The drawing under review shows one solid part. Ordinate dimensions are in mm from its lowest x, y, z. A direction names the side the tool comes from. Coordinates: 2 decimals unless noted, no trailing zeros. Write each loop counter-clockwise with the first axis right and the second up, starting at its lowest first coordinate (ties: lowest second). Pieces come first, ordered by that corner, then holes.
1) We need section C-C on x = 24. Write out the cut boundary in (y, z).
2) For the marked faces 1, 2 and 3, list the 3-axis set-ups (+Z, -Z, +X, -X, +Y, -Y) from which the entire face can be reached by the end or side of a thin tool; tool diameter is ignored.
3) We need section B-B on y = 4. Give the number of separate pieces and of enclosed holes in the cut face.
4) Insertion check: P1, Ø2.5, axis at x = 18, y = 3.125, coming from the -Z side; P2, Ø8, axis at x = 7, y = 14.5, coming from the +Z side; P3, Ø1.5, axis at x = 23.5, z = 6, coming from the -Y side; P4, Ø0.6, axis at y = 4, z = 21.5, coming from the -X side. Each pin has a flat end and moves straight along its axis. Give the tip position at first contact, or say it passes through.
5) To check wall thickness, follow line 1 along Y through (x, z) = (24, 0.55); line 2 along Y through (x, z) = (23, 19.5); line 3 along X through (y, z) = (10.5, 15). State the ranges of each line that lie inside material, in increasing order.
6) We need section A-A on x = 30. Write out the cut boundary in (y, z), then the cut area to 3 significant figures.
7) We need section D-D on y = 21. Write out the cut boundary in (x, z), then the cut area to 3 significant figures.
8) Mouldability with a two-part tool opening along Z and no side actions: class the marked faces 4, 5, 6 and 7 as pulls with the +Z half, pulls with the -Z half, needs draft (parallel to the pull), parting line crosses it, or undercut.
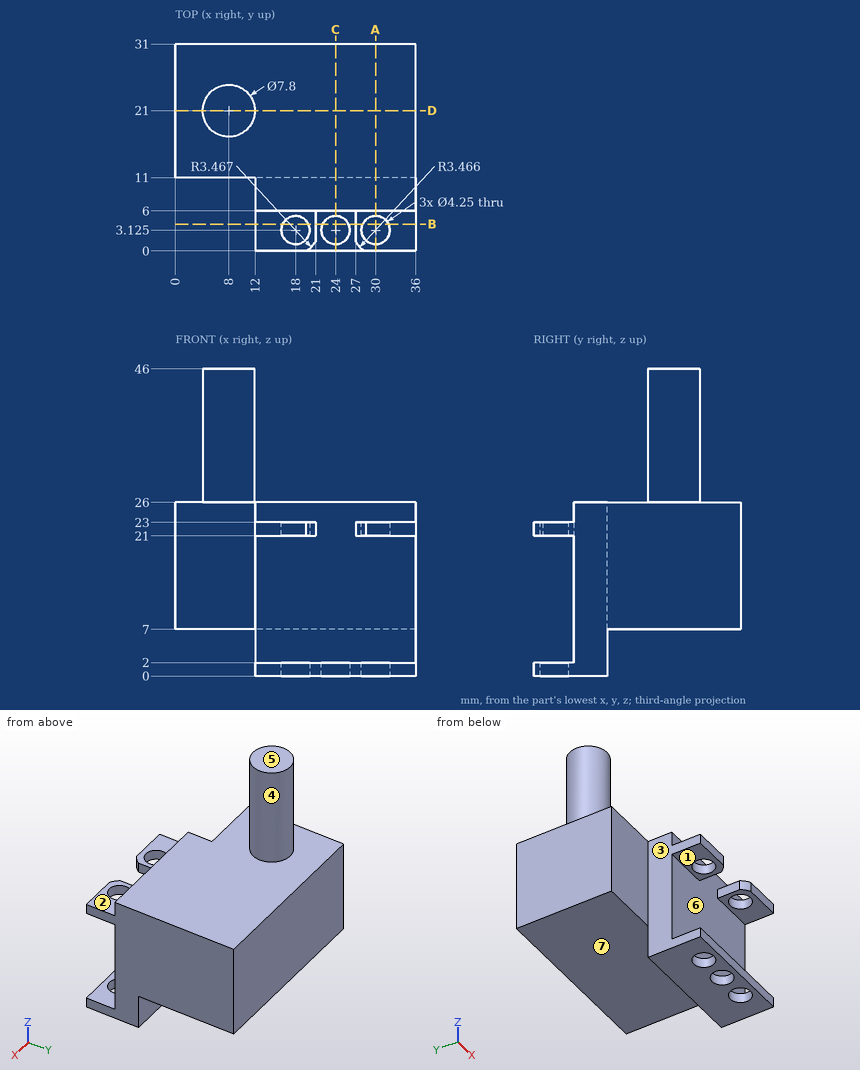
Result:
1. outline: (0, 0) - (1, 0) - (1, 2) - (0, 2) - close; (5.25, 0) - (11, 0) - (11, 7) - (31, 7) - (31, 26) - (6, 26) - (6, 2) - (5.25, 2) - close
2. face 1: +X, -X, -Y
2. face 2: +Z, +X, -X, -Y
2. face 3: +Z, -Z, -X, -Y
3. separate pieces: 8
3. enclosed holes: 0
4. P1: passes through
4. P2: stops at z = 46
4. P3: stops at y = 6
4. P4: stops at x = 12
5. line 1: y = 0 to 1, 5.25 to 11
5. line 2: y = 6 to 31
5. line 3: x = 12 to 36
6. outline: (0, 0) - (1, 0) - (1, 2) - (0, 2) - close; (0, 21) - (1, 21) - (1, 23) - (0, 23) - close; (5.25, 0) - (11, 0) - (11, 7) - (31, 7) - (31, 26) - (6, 26) - (6, 23) - (5.25, 23) - (5.25, 21) - (6, 21) - (6, 2) - (5.25, 2) - close
6. area: 517 mm2
7. outline: (0, 7) - (36, 7) - (36, 26) - (11.9, 26) - (11.9, 46) - (4.1, 46) - (4.1, 26) - (0, 26) - close
7. area: 840 mm2
8. face 4: needs draft
8. face 5: pulls with the +Z half
8. face 6: undercut
8. face 7: pulls with the -Z half
